Can you work these out from the drawing? Everything is in mm from the part's minimum corner. Round coordinates to 2 decimals unless told otherwise and drop trailing zeros. Loops run counter-clockwise (first coordinate to the right, second up) from the corner with the lowest first, then second, coordinate; pieces in that order, holes last. Notation, with made-up numbers: M 19,7.5 L 57,7.5 A4 ccw 57,11.5 Z; hole C 67.5,-7 d6. An arc over 180 degrees is marked long. Use a Markdown table: item, result.
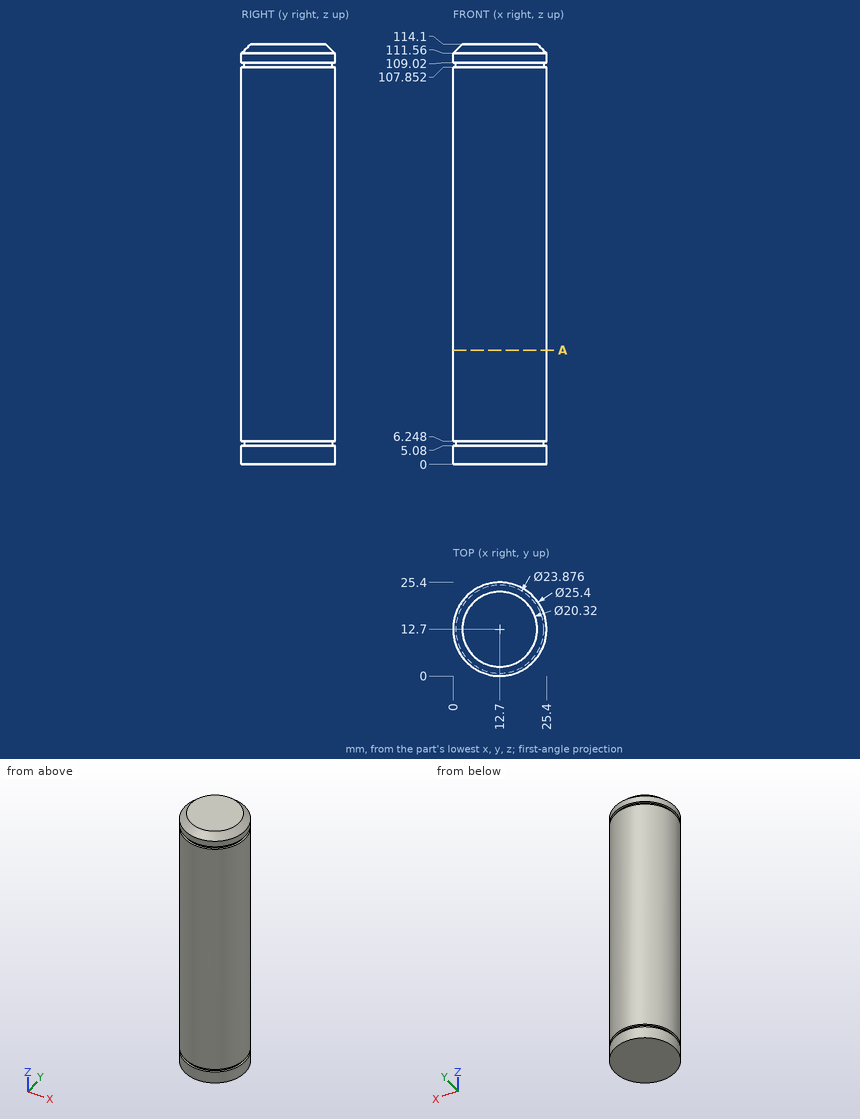
1. For pin 1 Ø4 at (x, z) = (22.5, 20) entering from -Y; pin 2 Ø2 at (y, z) = (14, 56) entering from +X, each with a flat end and sliding along its axis, tell me the tip position at first contact or that it passes through.
Answer sheet:
| item | result |
|---|---|
| pin 1 | y = 2.68 |
| pin 2 | x = 25.4 |
2. Imagine slicing it at A-A, the plane z = 31. Write out the boundary of the cut face in (x, y).
Answer sheet:
| item | result |
|---|---|
| outline | C 12.7,12.7 d25.4 |
3. I need wall thicknesses on probe 1 along Y at (x, z) = (13, 42); probe 2 along Y at (x, z) = (11, 50) (1 decimal). Which ranges of each line are inside material? Lowest first, please. Write a range as from..to.
Answer sheet:
| item | result |
|---|---|
| probe 1 | 0..25.4 |
| probe 2 | 0.1..25.3 |
